Source: CAD feature listing. Evaluate the final solid. Frame: model axes, mm. Face numbers are marked on the shaded views. A direction names the side the tool comes from. Give positions to 0.01 mm unless a question says otherwise; leave off trailing zeros. Order: outer loops, then holes, each group sorted by start corner. A loop starts at its lowest first (then second) coordinate and runs counter-clockwise, first axis right, second up. Notation, with made-up numbers: (25.5, 15.25) -> (35.5, 15.25) arc R19 ccw to (35.5, 23.25) -> close; hole circle Ø6 at (8, 89.25). An arc over 180 degrees is marked (long way). Use CSV: the item, a comma, the result in double quotes.
Autodesk Inventor part; units mm, degrees
ref_plane "YZ Plane" through (0, 0, 0) normal (1, 0, 0) x (0, 1, 0)
ref_plane "XZ Plane" through (0, 0, 0) normal (0, 1, 0) x (-1, 0, 0)
ref_plane "XY Plane" through (0, 0, 0) normal (0, 0, 1) x (1, 0, 0)
sketch "Sketch1" plane through (0, 0, 0) normal (0, 1, 0) x (-1, 0, 0)
  line L0 (61, 46.75) -> (-61, 46.75)
  line L1 (-61, 46.75) -> (-61, -46.75)
  line L2 (-61, -46.75) -> (61, -46.75)
  line L3 (61, -46.75) -> (61, 46.75)
  line L4 (-61, 46.75) -> (61, -46.75) construction
  line L5 (66, 51.75) -> (-66, 51.75)
  line L6 (-66, 51.75) -> (-66, -51.75)
  line L7 (-66, -51.75) -> (66, -51.75)
  line L8 (66, -51.75) -> (66, 51.75)
  line L9 (0, -51.75) -> (0, -46.75) construction
  line L10 (66, 0) -> (61, 0) construction
  line L11 (58, 45.75) -> (1, 45.75) construction
  line L12 (1, 45.75) -> (1, -43.25) construction
  line L13 (1, -43.25) -> (58, -43.25) construction
  line L14 (58, -43.25) -> (58, 45.75) construction
  line L15 (-4, 35.25) -> (-60, 35.25) construction
  line L16 (-60, 35.25) -> (-60, -45.75) construction
  line L17 (-60, -45.75) -> (-4, -45.75) construction
  line L18 (-4, -45.75) -> (-4, 35.25) construction
  line L19 (3, 10) -> (-1, 10)
  line L20 (-1, 10) -> (-1, -10)
  line L21 (-1, -10) -> (3, -10)
  line L22 (3, -10) -> (3, 10)
  line L23 (1, -43.25) -> (-4, -43.25) construction
  line L24 (0, 0) -> (3, 0) construction
  dimension "d2" = 5
  dimension "d7" = 57
  dimension "d8" = 89
  dimension "d9" = 3.5
  dimension "d10" = 1
  dimension "d11" = 56
  dimension "d12" = 5
  dimension "d13" = 3
  dimension "d14" = 1
  dimension "d15" = 81
  dimension "d16" = 1
  dimension "d17" = 4
  dimension "d18" = 20
  dimension "d37" = 60
extrude "Extrusion1" add sketch "Sketch1" against normal blind 5 contours L3 L2 L1 L0 | L8 L7 L6 L5 | L22 L21 L20 L19
extrude "Extrusion2" add sketch "Sketch1" along normal blind 75 contours L8 L7 L6 L5
extrude "Extrusion3" add sketch "Sketch1" along normal blind 10 contours L22 L21 L20 L19
fillet "Fillet1" radius 5 4 edges at (66, 35, 51.75) (-66, 35, 51.75) (-66, 35, -51.75) (66, 35, -51.75)
sketch "Sketch2" plane through (-66, -5, -46.75) normal (-1, 0, 0) x (0, 0, 1)
  circle A0 centre (10.9794, 28.8313) radius 8.5 construction
  circle A1 centre (35.9794, 28.8313) radius 8.5 construction
  circle A2 centre (11.25, 29) radius 8.5
  circle A3 centre (36.25, 29) radius 8.5
  line L0 (10.9794, 28.8313) -> (35.9794, 28.8313) construction
  line L1 (11.25, 29) -> (36.25, 29) construction
  line L2 (93.5, 0) -> (0, 0)
  point P0 (46.75, 5)
  point P1 (23.75, 29)
  point P2 (46.75, 0)
  dimension "d26" = 29
  dimension "d27" = 23
extrude "Extrusion4" cut sketch "Sketch2" against normal up to surface (5 mm away)
sketch "Sketch3" plane through (-66, -5, -46.75) normal (-1, 0, 0) x (0, 0, 1)
  line L0 (35.15, 65) -> (58.35, 65)
  line L1 (58.35, 65) -> (58.35, 41.8)
  line L2 (58.35, 41.8) -> (35.15, 41.8)
  line L3 (35.15, 41.8) -> (35.15, 65)
  line L4 (93.5, 0) -> (0, 0)
  line L5 (0, 80) -> (93.5, 80)
  point P0 (46.75, 5)
  point P1 (46.75, 0)
  point P2 (46.75, 41.8)
  dimension "d28" = 23.2
  dimension "d29" = 15
extrude "Extrusion5" cut sketch "Sketch3" against normal up to surface (5 mm away)
mirror "Mirror1" about plane through (0, 0, 0) normal (0, 0, 1) of "Extrusion4"
sketch "Sketch4" plane through (61, -5, -51.75) normal (0, 0, -1) x (-1, 0, 0)
  line L0 (25, 63) -> (97, 63)
  line L1 (97, 63) -> (97, 38)
  line L2 (97, 38) -> (25, 38)
  line L3 (25, 38) -> (25, 63)
  line L4 (0, 80) -> (122, 80)
  line L5 (24.8135, 37.7871) -> (96.8135, 37.7871)
  line L6 (96.8135, 37.7871) -> (96.8135, 62.7871)
  line L7 (96.8135, 62.7871) -> (24.8135, 62.7871)
  line L8 (24.8135, 62.7871) -> (24.8135, 37.7871)
  point P0 (61, 5)
  point P1 (61, 80)
  point P2 (61, 63)
  point P3 (25, 62.7871)
  point P4 (96.8135, 38)
  dimension "d32" = 72
  dimension "d33" = 25
  dimension "d34" = 17
extrude "Extrusion6" cut sketch "Sketch4" against normal up to surface (5 mm away) contours L7 L6 L2 L3
sketch "Sketch5" plane through (61, -5, -51.75) normal (0, 0, -1) x (-1, 0, 0)
  line L0 (41, 32) -> (61, 32)
  line L1 (61, 32) -> (61, 12)
  line L2 (61, 12) -> (41, 12)
  line L3 (41, 12) -> (41, 32)
  line L4 (0, 5) -> (0, 80)
  line L5 (122, 0) -> (0, 0)
  point P0 (61, 5)
  dimension "d38" = 20
  dimension "d39" = 41
  dimension "d40" = 12
extrude "Extrusion7" cut sketch "Sketch5" against normal up to surface (5 mm away)
sketch "Sketch6" plane through (66, -5, -46.75) normal (1, 0, 0) x (0, 0, -1)
  line L0 (-87.5, 19) -> (-75.5, 19)
  line L1 (-75.5, 19) -> (-75.5, 12)
  line L2 (-75.5, 12) -> (-87.5, 12)
  line L3 (-87.5, 12) -> (-87.5, 19)
  line L4 (0, 0) -> (-93.5, 0)
  line L5 (-93.5, 5) -> (-93.5, 80)
  point P0 (-46.75, 5)
  dimension "d43" = 12
  dimension "d44" = 7
  dimension "d45" = 12
  dimension "d46" = 6
extrude "Extrusion8" cut sketch "Sketch6" against normal up to surface (5 mm away)
properties part number "kucisteDonji"
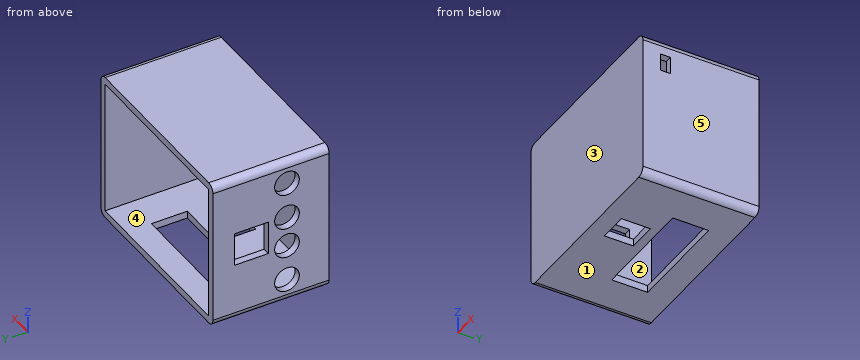
1. Section query D-D on z = -35.5. Return loops of the section in (x, y), plus the area to 4 significant figures.
Answer below:
outline,"(-66, -5) -> (66, -5) -> (66, 75) -> (61, 75) -> (61, 0) -> (-61, 0) -> (-61, 15.5) -> (-66, 15.5) -> close; (-66, 32.5) -> (-61, 32.5) -> (-61, 75) -> (-66, 75) -> close"
area,"1,325 mm²"
2. Mould query, pull axis X, two halves, no side actions, for the marked faces 3, 4 and 5. Classes: released by +X, released by -X, zero draft, split by the parting line, or undercut.
Answer below:
face 3,"zero draft"
face 4,"undercut"
face 5,"released by +X"
3. Access query for the marked faces 1 and 2. Directions: +Z, -Z, +X, -X, +Y, -Y. A direction counts if a zero-diameter tool reaches every point of the face in a straight line with its end or side. Return the directions, or none.
Answer below:
face 1,"-Z, +X, -X, +Y, -Y"
face 2,"+Y"
4. Section query A-A on y = 54.5. Return loops of the section in (x, z).
Answer below:
outline,"(-66, -46.75) arc R5 ccw to (-61, -51.75) -> (-35.81, -51.75) -> (-35.81, -46.75) -> (-61, -46.75) -> (-61, -11.6) -> (-66, -11.6) -> close; (-66, 11.6) -> (-61, 11.6) -> (-61, 46.75) -> (61, 46.75) -> (61, -46.75) -> (36, -46.75) -> (36, -51.75) -> (61, -51.75) arc R5 ccw to (66, -46.75) -> (66, 46.75) arc R5 ccw to (61, 51.75) -> (-61, 51.75) arc R5 ccw to (-66, 46.75) -> close"
5. Section query C-C on x = -6.5. Return loops of the section in (y, z), plus the area to 3 significant figures.
Answer below:
outline,"(-5, -51.75) -> (33, -51.75) -> (33, -46.75) -> (0, -46.75) -> (0, 46.75) -> (75, 46.75) -> (75, 51.75) -> (-5, 51.75) -> close; (57.79, -51.75) -> (75, -51.75) -> (75, -46.75) -> (57.79, -46.75) -> close"
area,"1,140 mm²"
6. Pin query (flat end, axial travel): P1, Ø12, axis at x = -49, z = 25.5, coming from the +Y side; P2, Ø2, axis at x = -1, z = -1.5, coming from the +Y side; P3, Ø4, axis at y = 15, z = -50, coming from the -X side; P4, Ø5.5, axis at x = -62.5, y = 47, coming from the +Z side. Return the tip coordinate at first contact, or that it passes through.
Answer below:
P1,"stops at y = 0"
P2,"stops at y = 10"
P3,"stops at x = -65.84"
P4,"stops at z = 51.75"
7. Section query B-B on y = 24. Count the separate pieces of the cut face and the enclosed holes in it, plus the area to 3 significant figures.
Answer below:
separate pieces,"5"
enclosed holes,"0"
area,"1,790 mm²"
8. Ray query, line 1 along X through (y, z) = (57, 27.5); line 2 along Y through (x, z) = (-64, -10); line 3 along Z through (x, y) = (-36, 14.5). Return the intervals inside material, ascending.
Answer below:
line 1,"x = -66 to -61, 61 to 66"
line 2,"y = -5 to 15.51, 32.49 to 36.8, 60 to 75"
line 3,"z = -51.75 to -46.75, 46.75 to 51.75"
